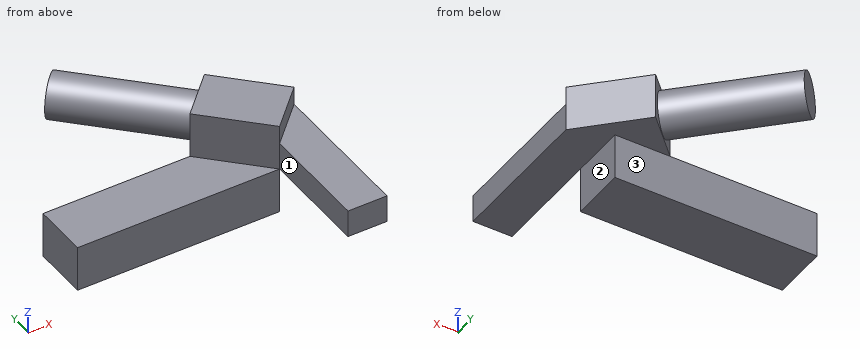
from build123d import *

# Parameters (mm, degrees)
F0_W     = 220
F0_H     = 60
F1_DEPTH = 50
F3_DEPTH = 50
F4_DEPTH = 25
F5_R     = 20
F6_DEPTH = 60
F6_TAPER = -3
F7_DEPTH = 199
F9_DEPTH = 30


with BuildPart() as f1:
    # F0 (on Top) → F1 (new body)
    with BuildSketch(Plane.XY):
        Rectangle(F0_W, F0_H)
    extrude(amount=F1_DEPTH)

    # F2 (on face) → F3 (join)
    with BuildSketch(Plane.XY.offset(50)):
        Polygon((50, 30), (110, -30), (152.4264068712, 12.4264068712), (92.4264068712, 72.4264068712), align=None)
    extrude(amount=F3_DEPTH)

    # F2 (on face) → F4 (join)
    with BuildSketch(Plane.XY.offset(50)):
        Polygon((50, 30), (110, -30), (152.4264068712, 12.4264068712), (92.4264068712, 72.4264068712), align=None)
    extrude(amount=F4_DEPTH)

    # F5 (on face) → F6 (cut)
    with BuildSketch(Plane(origin=(10, -10, 0), x_dir=(-0.7071067812, -0.7071067812, 0), z_dir=(-0.7071067812, 0.7071067812, 0))):
        with Locations((-86.5685424949, 75)):
            Circle(F5_R)
    extrude(amount=-F6_DEPTH, taper=F6_TAPER, mode=Mode.SUBTRACT)

    # F7 (add): a face of the model
    f7_faces = [f1.faces().sort_by_distance(p)[0] for p in [
        (113.6396103068, 8.7867965644, 75),
    ]]
    extrude(f7_faces, amount=F7_DEPTH)

    # F8 (on face) → F9 (join)
    with BuildSketch(Plane.XY.offset(50)):
        Polygon((152.4264068712, 12.4264068712), (110, -30), (110, -148.6592590809), (152.4264068712, -148.6592590809), align=None)
    extrude(amount=F9_DEPTH)


solid = f1.part
Geometry check sheet. Reference: the model listing, model coordinates, mm. Face numbers are marked on the shaded views. A direction names the side the tool comes from. Coordinates: 2 decimals unless noted, no trailing zeros. Order: outer loops, then holes, each group sorted by start corner. A loop starts at its lowest first (then second) coordinate and runs counter-clockwise, first axis right, second up. Notation, with made-up numbers: M 54,16 L 93,16 A33 cw 93,52 Z; hole C 21,50.25 d5. An arc over 180 degrees is marked long. Use CSV: the item, a comma, the result in double quotes.
Item 1: Cross-section at C-C on x = 123.5. Record the cut outline in (y, z), then the cut area to 3 significant figures.
Returned:
outline,"M -148.66,50 L 41.35,50 L 41.35,100 L -16.5,100 L -16.5,80 L -148.66,80 Z"
area,"6,860 mm2"
Item 2: Cross-section at A-A on y = -21. Record the cut outline in (x, z).
Returned:
outline,"M -110,0 L 110,0 L 110,50 L 152.43,50 L 152.43,80 L 119,80 L 119,100 L 101,100 L 101,50 L -110,50 Z"
Item 3: Tool access check on the marked faces 1, 2 and 3. Record the directions out of +Z, -Z, +X, -X, +Y, -Y that give a thin tool (end or side, any length) a straight path to the whole face; none if there is none.
Returned:
face 1,"+Z, -Z, -X, -Y"
face 2,"-Z, +X, +Y, -Y"
face 3,"-Z, +X, -X, +Y"
Item 4: Cross-section at B-B on z = 70. Record the cut outline in (x, y), then the cut area to 3 significant figures.
Returned:
outline,"M -43.05,133.52 L 55.23,35.23 L 50,30 L 110,-30 L 110,-148.66 L 152.43,-148.66 L 152.43,12.43 L 92.43,72.43 L 87.19,67.19 L -11.1,165.48 Z"
area,"17,300 mm2"
Item 5: Gauge pin test, flat ends, axial feed: pin 1 Ø1 at (y, z) = (-48.5, 77.5) entering from -X; pin 2 Ø15 at (x, z) = (-1, 15.5) entering from -Y; pin 3 Ø3 at (y, z) = (18.5, 78.5) entering from -X. Record the tip position at first contact, or that the pin passes through.
Returned:
pin 1,"stops at x = 110"
pin 2,"stops at y = -30"
pin 3,"stops at x = 60"
Item 6: Cross-section at D-D on z = 43. Record the cut outline in (x, y).
Returned:
outline,"M -110,-30 L 110,-30 L 110,30 L -110,30 Z"
Item 7: Thickness scan on line 1 along Z through (x, y) = (-81, 2); line 2 along Y through (x, z) = (109, 24.5); line 3 along X through (y, z) = (63, 92). Record the ranges inside material, lowest first.
Returned:
line 1,"z = 0 to 50"
line 2,"y = -30 to 30"
line 3,"x = 37.22 to 81.64, 83 to 101.85"
